Geometry: final body of the model. Coordinates: model frame, mm. Face numbers are marked on the shaded views. A direction names the side the tool comes from. Round coordinates to 2 decimals unless told otherwise and drop trailing zeros. Loops run counter-clockwise (first coordinate to the right, second up) from the corner with the lowest first, then second, coordinate; pieces in that order, holes last. Notation, with made-up numbers: M 26,-35.5 L 76,-35.5 A14 ccw 76,-31.5 Z; hole C 10,46 d1. An arc over 180 degrees is marked long. Return JSON: item names as keys, results as strings.
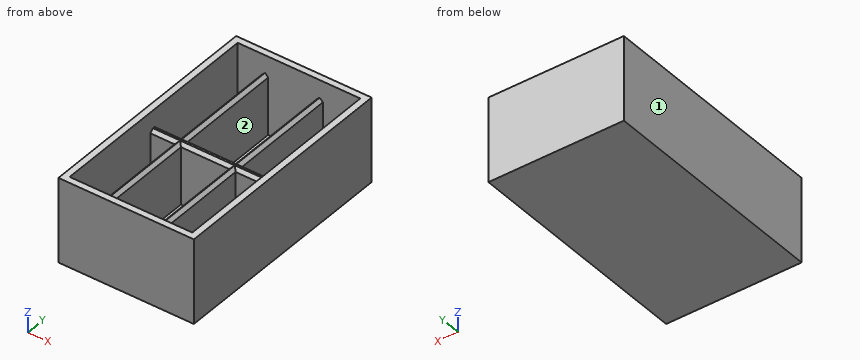
from build123d import *

# Parameters (mm, degrees)
F0_W     = 2.4
F0_H     = 40
F0_H_2   = 3.2
F1_DEPTH = 31.6
F0_W_2   = 9
F0_W_3   = 18
F0_W_4   = 14
F2_DEPTH = 2.4
F3_DEPTH = 25
F4_SIZE  = 1.19999


# Not quite as in the source:
# - a fillet or chamfer is up to 0.001 mm smaller than in the source, because OpenCascade refuses the exact size


with BuildPart() as f1:
    # F0 (on Top) → F1 (new body)
    with BuildSketch(Plane.XY):
        Polygon((-9.4000064151, 44), (-60.0000064151, 44), (-60.0000064151, -44), (-9.4000064151, -44), (-9.4000064151, -41.6), (-11.8000064151, -41.6), (-25.8000064151, -41.6), (-28.2000064151, -41.6), (-46.2000064151, -41.6), (-48.6000064151, -41.6), (-57.6000064151, -41.6), (-57.6000064151, -1.6), (-57.6000064151, 1.6), (-57.6000064151, 41.6), (-48.6000064151, 41.6), (-46.2000064151, 41.6), (-28.2000064151, 41.6), (-25.8000064151, 41.6), (-11.8000064151, 41.6), (-9.4000064151, 41.6), align=None)
        with Locations((-10.6000064151, 21.6)):
            Rectangle(F0_W, F0_H)
        with Locations((-10.6000064151, 0)):
            Rectangle(F0_W, F0_H_2)
        with Locations((-10.6000064151, -21.6)):
            Rectangle(F0_W, F0_H)
    extrude(amount=F1_DEPTH)

    # F0 (on Top) → F2 (join)
    with BuildSketch(Plane.XY):
        with Locations((-53.1000064151, 21.6)):
            Rectangle(F0_W_2, F0_H)
        with Locations((-53.1000064151, 0)):
            Rectangle(F0_W_2, F0_H_2)
        with Locations((-53.1000064151, -21.6)):
            Rectangle(F0_W_2, F0_H)
        with Locations((-37.2000064151, 21.6)):
            Rectangle(F0_W_3, F0_H)
        with Locations((-37.2000064151, 0)):
            Rectangle(F0_W_3, F0_H_2)
        with Locations((-37.2000064151, -21.6)):
            Rectangle(F0_W_3, F0_H)
        with Locations((-18.8000064151, 21.6)):
            Rectangle(F0_W_4, F0_H)
        with Locations((-18.8000064151, 0)):
            Rectangle(F0_W_4, F0_H_2)
        with Locations((-18.8000064151, -21.6)):
            Rectangle(F0_W_4, F0_H)
    extrude(amount=F2_DEPTH)

    # F0 (on Top) → F3 (join)
    with BuildSketch(Plane.XY):
        Polygon((-9.4000064151, 44), (-60.0000064151, 44), (-60.0000064151, -44), (-9.4000064151, -44), (-9.4000064151, -41.6), (-11.8000064151, -41.6), (-25.8000064151, -41.6), (-28.2000064151, -41.6), (-46.2000064151, -41.6), (-48.6000064151, -41.6), (-57.6000064151, -41.6), (-57.6000064151, -1.6), (-57.6000064151, 1.6), (-57.6000064151, 41.6), (-48.6000064151, 41.6), (-46.2000064151, 41.6), (-28.2000064151, 41.6), (-25.8000064151, 41.6), (-11.8000064151, 41.6), (-9.4000064151, 41.6), align=None)
        with Locations((-10.6000064151, 21.6)):
            Rectangle(F0_W, F0_H)
        with Locations((-10.6000064151, -21.6)):
            Rectangle(F0_W, F0_H)
        with Locations((-10.6000064151, 0)):
            Rectangle(F0_W, F0_H_2)
        with Locations((-53.1000064151, 0)):
            Rectangle(F0_W_2, F0_H_2)
        with Locations((-47.4000064151, 0)):
            Rectangle(F0_W, F0_H_2)
        with Locations((-47.4000064151, 21.6)):
            Rectangle(F0_W, F0_H)
        with Locations((-47.4000064151, -21.6)):
            Rectangle(F0_W, F0_H)
        with Locations((-37.2000064151, 0)):
            Rectangle(F0_W_3, F0_H_2)
        with Locations((-27.0000064151, 21.6)):
            Rectangle(F0_W, F0_H)
        with Locations((-27.0000064151, 0)):
            Rectangle(F0_W, F0_H_2)
        with Locations((-18.8000064151, 0)):
            Rectangle(F0_W_4, F0_H_2)
        with Locations((-27.0000064151, -21.6)):
            Rectangle(F0_W, F0_H)
    extrude(amount=F3_DEPTH)

    # F4 (size 1.2 in the source; OpenCascade refuses exactly that, so slightly less here)
    f4_edges = [f1.edges().sort_by_distance(p)[0] for p in [
        (-53.100006, 1.6, 25),
        (-53.100006, -1.6, 25),
        (-46.200006, -21.6, 25),
        (-48.600006, -21.6, 25),
        (-48.600006, 21.6, 25),
        (-46.200006, 21.6, 25),
        (-37.200006, 1.6, 25),
        (-37.200006, -1.6, 25),
        (-28.200006, -21.6, 25),
        (-25.800006, -21.6, 25),
        (-18.800006, -1.6, 25),
        (-18.800006, 1.6, 25),
        (-25.800006, 21.6, 25),
        (-28.200006, 21.6, 25),
    ]]
    chamfer(f4_edges, length=F4_SIZE)


solid = f1.part
Q1. Pin query (flat end, axial travel): pin 1 (4.5 mm diameter, centred on x = -54.5, y = -26.5, fed in from +Z); pin 2 (20 mm diameter, centred on x = -36, y = 16, fed in from +Z). Return the tip coordinate at first contact, or that it passes through.
Determined:
{"pin 1": "stops at z = 2.4", "pin 2": "stops at z = 25"}
Q2. Section query A-A (z = 22). Output: boundary loops of the cut face in (x, y).
Determined:
{"outline": "M -60,-44 L -9.4,-44 L -9.4,44 L -60,44 Z; hole M -57.6,-41.6 L -48.6,-41.6 L -48.6,-1.6 L -57.6,-1.6 Z; hole M -57.6,1.6 L -48.6,1.6 L -48.6,41.6 L -57.6,41.6 Z; hole M -46.2,-41.6 L -28.2,-41.6 L -28.2,-1.6 L -46.2,-1.6 Z; hole M -46.2,1.6 L -28.2,1.6 L -28.2,41.6 L -46.2,41.6 Z; hole M -25.8,-41.6 L -11.8,-41.6 L -11.8,-1.6 L -25.8,-1.6 Z; hole M -25.8,1.6 L -11.8,1.6 L -11.8,41.6 L -25.8,41.6 Z"}
Q3. Section query C-C (z = 28.5). Output: boundary loops of the cut face in (x, y).
Determined:
{"outline": "M -60,-44 L -9.4,-44 L -9.4,44 L -60,44 Z; hole M -57.6,-41.6 L -11.8,-41.6 L -11.8,41.6 L -57.6,41.6 Z"}
Q4. Reachability of the marked faces 1 and 2 from +Z, -Z, +X, -X, +Y, -Y: full face, straight path, thin tool, end or side. Return the list, or none.
Determined:
{"face 1": "+Z, -Z, -X, +Y, -Y", "face 2": "+Z"}
Q5. Material intervals for L1, parallel to X at y = -28.5, z = 7.5; L2, parallel to Y at x = -36, z = 15.5; L3, parallel to X at y = 26.5, z = 28.5, sorted ascending.
Determined:
{"L1": "x = -60 to -57.6, -48.6 to -46.2, -28.2 to -25.8, -11.8 to -9.4", "L2": "y = -44 to -41.6, -1.6 to 1.6, 41.6 to 44", "L3": "x = -60 to -57.6, -11.8 to -9.4"}
Q6. Section query B-B (x = -17). Output: boundary loops of the cut face in (y, z), plus the area to 3 significant figures.
Determined:
{"outline": "M -44,0 L 44,0 L 44,31.6 L 41.6,31.6 L 41.6,2.4 L 1.6,2.4 L 1.6,23.8 L 0.4,25 L -0.4,25 L -1.6,23.8 L -1.6,2.4 L -41.6,2.4 L -41.6,31.6 L -44,31.6 Z", "area": "422 mm^2"}
